Verification items for the finished model (mm, model axes). A direction names the side the tool comes from. Give positions to 0.01 mm unless a question says otherwise; leave off trailing zeros. Order: outer loops, then holes, each group sorted by start corner. A loop starts at its lowest first (then second) coordinate and runs counter-clockwise, first axis right, second up. Notation, with made-up numbers: (42, 59) - (65, 59) arc R7 cw to (65, 68) - close; hole circle Ø4 at (-29, -36). An arc over 180 degrees is marked (long way). Answer as a JSON object with one key per item and string values. Group by question number.
(1) Section check C-C (y = -5). Record the boundary of the cut face in (x, z).
(2) Section check D-D (x = 39.5). Record the boundary of the cut face in (y, z).
(3) Thickness scan on line 1 (X direction, y = 1.5, z = -28); line 2 (Z direction, x = 67.5, y = 4); line 3 (Z direction, x = 23, y = -6.5). Record the ranges inside material, lowest first.
(4) Section check A-A (z = -46.5). Record the boundary of the cut face in (x, y).
(5) Depth check by flat-ended pin: pin 1 Ø4 at (x, y) = (12, -19.5) entering from +Z; pin 2 Ø9.5 at (y, z) = (-5, -38) entering from +X; pin 3 Ø2 at (x, z) = (36.5, -12.5) entering from +Y; pin 4 Ø1.5 at (x, z) = (8.5, -16.5) entering from -Y. Enter the tip coordinate at first touch or a pass-through.
(6) Section check B-B (x = 67.5). Record the boundary of the cut face in (y, z).
(7) Access from +Z, -Z, +X, -X, +Y, -Y to the whole of each face (thin tool, end or side, straight path). Record for faces 5 (the face through (25, -10, -51)), 6 (the face through (0, -16, -28)).
(8) Mould release check, pull along X, two halves, no side actions. Record for faces 1 (the face through (5, -19, -28)), 2 (the face through (2.46, -2.97, -20.21)), 3 (the face through (65.79, 2.46, -12.88)), 4 (the face through (56.957, 2.465, -28.651)): +X half, -X half, draft (parallel to the pull), parting line (faces both ways), or undercut.
```python
from build123d import *

# Parameters (mm, degrees)
SKETCH_1_W          = 74
SKETCH_1_H          = 56
SKETCH_1_R          = 2.5
SKETCH_1_R_2        = 5
SKETCH_1_R_3        = 1.75
EXTRUDE_1_DEPTH     = 5
EXTRUDE_2_DEPTH     = 38
CUT_EXTRUDE_1_REACH = 102.28
SKETCH_4_R          = 3
CUT_EXTRUDE_2_DEPTH = 5


with BuildPart() as part:
    # Эскиз1 → Бобышка-Вытянуть1 (new body)
    with BuildSketch(Plane(origin=(0, 0, 0), x_dir=(1, 0, 0), z_dir=(0, 1, 0))):
        with Locations((37, 28)):
            Rectangle(SKETCH_1_W, SKETCH_1_H)
        with Locations(Location((16, 46.5, 0), (0, 0, 270))):
            Circle(SKETCH_1_R, mode=Mode.SUBTRACT)
        with Locations(Location((16, 9.5, 0), (0, 0, 270))):
            Circle(SKETCH_1_R, mode=Mode.SUBTRACT)
        with Locations(Location((52, 46.5, 0), (0, 0, 270))):
            Circle(SKETCH_1_R, mode=Mode.SUBTRACT)
        with Locations(Location((52, 9.5, 0), (0, 0, 270))):
            Circle(SKETCH_1_R, mode=Mode.SUBTRACT)
        with Locations(Location((52, 28, 0), (0, 0, 270))):
            Circle(SKETCH_1_R_2, mode=Mode.SUBTRACT)
        with Locations(Location((67.5, 12.5, 0), (0, 0, 270))):
            Circle(SKETCH_1_R_3, mode=Mode.SUBTRACT)
        with Locations(Location((67.5, 43.5, 0), (0, 0, 270))):
            Circle(SKETCH_1_R_3, mode=Mode.SUBTRACT)
        with Locations(Location((36.5, 43.5, 0), (0, 0, 270))):
            Circle(SKETCH_1_R_3, mode=Mode.SUBTRACT)
        with Locations(Location((36.5, 12.5, 0), (0, 0, 270))):
            Circle(SKETCH_1_R_3, mode=Mode.SUBTRACT)
        with Locations(Location((16, 28, 0), (0, 0, 270))):
            Circle(SKETCH_1_R_2, mode=Mode.SUBTRACT)
    extrude(amount=EXTRUDE_1_DEPTH)

    # Эскиз2 → Бобышка-Вытянуть2 (add)
    with BuildSketch(Plane(origin=(0, 0, 0), x_dir=(-1, 0, 0), z_dir=(0, -1, 0))):
        Polygon((-74, 0), (0, 0), (0, 56), (-74, 56), (-74, 51), (-5, 51), (-5, 5), (-74, 5), align=None)
    extrude(amount=EXTRUDE_2_DEPTH)

    # Вырез-Вытянуть1: up to this face of the body (flat: up to its plane)
    cut_extrude_1_end = Plane(part.part.faces().sort_by_distance((37, -16.5, -56))[0])
    # Эскиз3 → Вырез-Вытянуть1 (cut, up to the picked face)
    with BuildSketch(Plane.XY, mode=Mode.PRIVATE) as cut_extrude_1_sk1:
        Polygon((5, -38), (74, 0), (74, -38), align=None)
    cut_extrude_1_tool1 = split(extrude(cut_extrude_1_sk1.sketch, amount=-CUT_EXTRUDE_1_REACH, mode=Mode.PRIVATE), bisect_by=cut_extrude_1_end, keep=Keep.BOTH, mode=Mode.PRIVATE)
    add(cut_extrude_1_tool1.solids().sort_by(Axis((51, -25.333333, 0), (0, 0, -1)))[0], mode=Mode.SUBTRACT)

    # Эскиз4 → Вырез-Вытянуть2 (cut)
    with BuildSketch(Plane.ZY):
        with Locations((-18, -25)):
            Circle(SKETCH_4_R)
        with Locations((-18, -5)):
            Circle(SKETCH_4_R)
        with Locations((-38, -5)):
            Circle(SKETCH_4_R)
        with Locations((-38, -25)):
            Circle(SKETCH_4_R)
    extrude(amount=-CUT_EXTRUDE_2_DEPTH, mode=Mode.SUBTRACT)


solid = part.part
```
Solutions:
{
 "1": {"outline": "(0, -56) - (64.92, -56) - (64.92, -51) - (5, -51) - (5, -41) - (0, -41) - close; (0, -35) - (5, -35) - (5, -21) - (0, -21) - close; (0, -15) - (5, -15) - (5, -5) - (64.92, -5) - (64.92, 0) - (0, 0) - close"},
 "2": {"outline": "(-19, -56) - (5, -56) - (5, 0) - (-19, 0) - (-19, -5) - (0, -5) - (0, -51) - (-19, -51) - close"},
 "3": {"line 1": "x = 0 to 11, 21 to 47, 57 to 74", "line 2": "z = -56 to -45.25, -41.75 to -14.25, -10.75 to 0", "line 3": "z = -56 to -51, -5 to 0"},
 "4": {"outline": "(0, -38) - (5, -38) - (5, 0) - (13.5, 0) - (13.5, 5) - (0, 5) - close; (18.5, 0) - (49.5, 0) - (49.5, 5) - (18.5, 5) - close; (54.5, 0) - (74, 0) - (74, 5) - (54.5, 5) - close"},
 "5": {"pin 1": "stops at z = 0", "pin 2": "stops at x = 5", "pin 3": "passes through", "pin 4": "stops at y = 0"},
 "6": {"outline": "(-3.58, -56) - (5, -56) - (5, -45.25) - (0, -45.25) - (0, -51) - (-3.58, -51) - close; (-3.58, -5) - (0, -5) - (0, -10.75) - (5, -10.75) - (5, 0) - (-3.58, 0) - close; (0, -41.75) - (5, -41.75) - (5, -14.25) - (0, -14.25) - close"},
 "7": {"face 5": "+X, -Y", "face 6": "+Z, -Z, -X, +Y, -Y"},
 "8": {"face 1": "+X half", "face 2": "draft", "face 3": "undercut", "face 4": "undercut"}
}
